Job drawing, mm, ordinate dimensions from the low corner. One solid piece. A direction names the side the tool comes from. Round coordinates to 2 decimals unless told otherwise and drop trailing zeros. Loops run counter-clockwise (first coordinate to the right, second up) from the corner with the lowest first, then second, coordinate; pieces in that order, holes last. Notation, with made-up numbers: M -22,31.25 L -4,31.25 A15 ccw -4,50.25 Z; hole C 62,69.5 d2. An arc over 180 degrees is marked long. Put each result on its own line as item: value. Start each with the question number.
1) Probe line 1 along Z through (x, y) = (4.5, 7.5); line 2 along Y through (x, z) = (6.25, 4.75). List the from-to ranges inside material, lowest first.
2) Drop flat-ended pins along their axis: pin 1 Ø6 at (y, z) = (11, 7) entering from +X; pin 2 Ø1 at (x, y) = (8.5, 11) entering from +Z; pin 3 Ø2.5 at (x, z) = (9.5, 9.5) entering from -Y. Give the stop position or say it passes through.
3) Slice it at A-A on x = 4.5. Give the cut face in (y, z), then the cut area to 3 significant figures.
4) Which spindle directions (+Z, -Z, +X, -X, +Y, -Y) get a long thin tool onto all of the face, cutting with end or side? Do the marked faces 1 and 2. Say none if no direction does.
5) Slice it at B-B on y = 13.5. Give the cut face in (x, z), then the cut area to 3 significant figures.
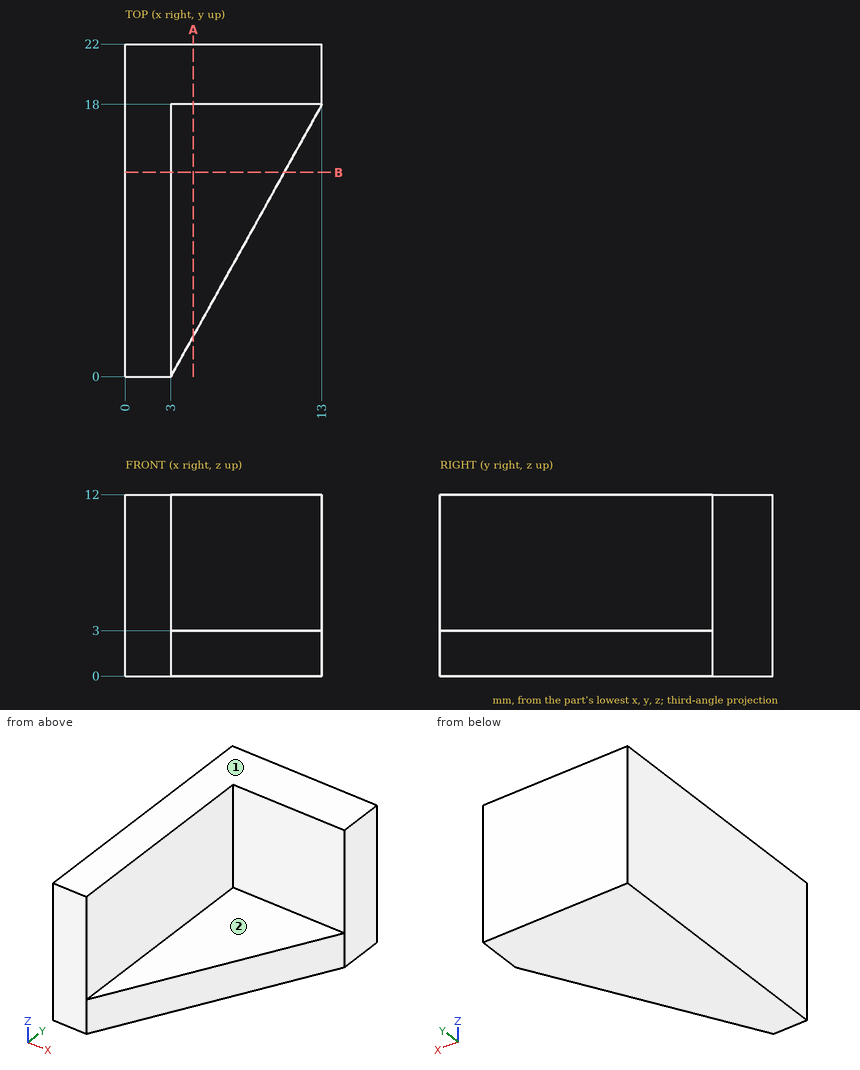
Recorded:
1. line 1: z = 0 to 3
1. line 2: y = 18 to 22
2. pin 1: stops at x = 3
2. pin 2: stops at z = 3
2. pin 3: stops at y = 18
3. outline: M 2.7,0 L 22,0 L 22,12 L 18,12 L 18,3 L 2.7,3 Z
3. area: 93.9 mm2
4. face 1: +Z, +X, -X, +Y, -Y
4. face 2: +Z, +X, -Y
5. outline: M 0,0 L 10.5,0 L 10.5,3 L 3,3 L 3,12 L 0,12 Z
5. area: 58.5 mm2
